Part model, mm, in its own coordinate system. Round coordinates to 2 decimals unless told otherwise and drop trailing zeros. Write each loop counter-clockwise with the first axis right and the second up, starting at its lowest first coordinate (ties: lowest second). Pieces come first, ordered by that corner, then holes. Notation, with made-up numbers: M 12.25,58.25 L 32.25,58.25 A15 cw 32.25,75.25 Z; hole C 60,-17.5 d9. An arc over 180 degrees is marked long. One line per question, with ' | ' between items. Start each with the question number.
1) Saw through at B-B (y = 0). List the corners of the cut face in (x, z).
2) Wall check: probe 1 along Z at (x, y) = (48, 24); probe 2 along X at (y, z) = (42.5, 4.5); probe 3 along X at (y, z) = (0.5, 1.75). Give the ranges that are in metal, low to high. Write a range as [from, to].
3) Drop flat-ended pins along their axis: pin 1 Ø1.5 at (y, z) = (27.5, -1.5) entering from +X; pin 2 Ø1.5 at (y, z) = (-17, 3.5) entering from +X; pin 3 Ø1 at (x, z) = (-48.5, 4) entering from -Y; pin 4 Ø4 at (y, z) = (-36, -1.5) entering from +X. Give the stop position or say it passes through.
4) Saw through at C-C (z = 2.5). List the corners of the cut face in (x, y) (3 decimals), plus the area to 3 significant figures.
5) Saw through at D-D (y = -15.5). List the corners of the cut face in (x, z), plus the area to 3 significant figures.
6) Saw through at A-A (x = 13.5). List the corners of the cut face in (y, z), plus the area to 3 significant figures.
```python
from build123d import *

# Parameters (mm, degrees)
BOSS_EXTRUDE1_DEPTH                               = 6
CSK_FOR_8_FLAT_HEAD_MACHINE_SCREW_100_D           = 4.3053
CSK_FOR_8_FLAT_HEAD_MACHINE_SCREW_100_CSINK_D     = 8.4328
CSK_FOR_8_FLAT_HEAD_MACHINE_SCREW_100_CSINK_ANGLE = 100
SKETCH5_R                                         = 1.905
BOSS_EXTRUDE2_DEPTH                               = 2.5
FILLET1_R                                         = 10
CUT_EXTRUDE1_DEPTH                                = 3.8


with BuildPart() as part:
    # Sketch1 → Boss-Extrude1 (new body)
    with BuildSketch(Plane.XY):
        with BuildLine():
            Line((-26.167728216, 59.5), (26.167728216, 59.5))
            ThreePointArc((26.167728216, 59.5), (65, 0), (26.167728216, -59.5))
            Line((26.167728216, -59.5), (-26.167728216, -59.5))
            ThreePointArc((-26.167728216, -59.5), (-65, 0), (-26.167728216, 59.5))
        make_face()
        with BuildLine():
            Line((-23.650581388, 48.1), (23.650581388, 48.1))
            ThreePointArc((23.650581388, 48.1), (53.6, 0), (23.650581388, -48.1))
            Line((23.650581388, -48.1), (-23.650581388, -48.1))
            ThreePointArc((-23.650581388, -48.1), (-53.6, 0), (-23.650581388, 48.1))
        make_face(mode=Mode.SUBTRACT)
    extrude(amount=BOSS_EXTRUDE1_DEPTH)

    # CSK for #8 Flat Head Machine Screw (100)1 (through all)
    with Locations(Plane.XY.offset(6)):
        with Locations((0, 0), (41.985, 41.985), (-41.985, -41.985), (-41.985, 41.985), (41.985, -41.985)):
            CounterSinkHole(CSK_FOR_8_FLAT_HEAD_MACHINE_SCREW_100_D / 2, CSK_FOR_8_FLAT_HEAD_MACHINE_SCREW_100_CSINK_D / 2, counter_sink_angle=CSK_FOR_8_FLAT_HEAD_MACHINE_SCREW_100_CSINK_ANGLE)

    # Sketch5 → Boss-Extrude2 (add)
    with BuildSketch(Plane(origin=(0, 0, 0), x_dir=(-1, 0, 0), z_dir=(0, 0, -1))):
        with Locations(Location((-59.2455, 0, 0), (0, 0, 180))):
            Circle(SKETCH5_R)
        with Locations(Location((59.2455, 0, 0), (0, 0, 180))):
            Circle(SKETCH5_R)
    extrude(amount=BOSS_EXTRUDE2_DEPTH)

    # Fillet1
    fillet1_edges = [part.edges().sort_by_distance(p)[0] for p in [
        (26.167728216, -59.5, 3),
        (-26.167728216, -59.5, 3),
        (-26.167728216, 59.5, 3),
        (26.167728216, 59.5, 3),
    ]]
    fillet(fillet1_edges, radius=FILLET1_R)

    # Sketch6 → Cut-Extrude1 (cut)
    with BuildSketch(Plane(origin=(0, 0, 0), x_dir=(-1, 0, 0), z_dir=(0, 0, -1))):
        with BuildLine():
            Line((22.912878475, 50), (-22.912878475, 50))
            ThreePointArc((-22.912878475, 50), (-55, 0), (-22.912878475, -50))
            Line((-22.912878475, -50), (22.912878475, -50))
            ThreePointArc((22.912878475, -50), (55, 0), (22.912878475, 50))
        make_face()
    extrude(amount=-CUT_EXTRUDE1_DEPTH, mode=Mode.SUBTRACT)


solid = part.part
```
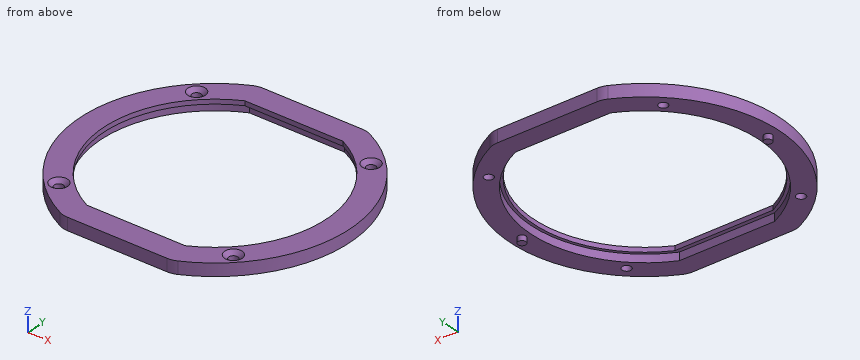
Answer key:
1) outline: M -65,0 L -61.15,0 L -61.15,-2.5 L -57.34,-2.5 L -57.34,0 L -55,0 L -55,3.8 L -53.6,3.8 L -53.6,6 L -65,6 Z; M 53.6,3.8 L 55,3.8 L 55,0 L 57.34,0 L 57.34,-2.5 L 61.15,-2.5 L 61.15,0 L 65,0 L 65,6 L 53.6,6 Z
2) probe 1: z = [3.8, 6] | probe 2: x = [-49.18, -44.36], [-39.61, -32.66], [32.66, 39.61], [44.36, 49.18] | probe 3: x = [-65, -55], [55, 65]
3) pin 1: passes through | pin 2: stops at x = 62.94 | pin 3: stops at y = -43.83 | pin 4: stops at x = 54.98
4) outline: M -28.333,-58.5 A10 ccw -23.974,-59.5 L 23.974,-59.5 A10 ccw 28.333,-58.5 A65 ccw 28.333,58.5 A10 ccw 23.974,59.5 L -23.974,59.5 A10 ccw -28.333,58.5 A65 ccw Z; hole C -41.985,-41.985 d4.305; hole C -41.985,41.985 d4.305; hole M -22.913,-50 L 22.913,-50 A55 ccw 22.913,50 L -22.913,50 A55 ccw Z; hole C 41.985,-41.985 d4.305; hole C 41.985,41.985 d4.305 | area: 3,630 mm2
5) outline: M -63.12,0 L -52.77,0 L -52.77,3.8 L -51.31,3.8 L -51.31,6 L -63.12,6 Z; M 51.31,3.8 L 52.77,3.8 L 52.77,0 L 63.12,0 L 63.12,6 L 51.31,6 Z | area: 131 mm2
6) outline: M -59.5,0 L -50,0 L -50,3.8 L -48.1,3.8 L -48.1,6 L -59.5,6 Z; M 48.1,3.8 L 50,3.8 L 50,0 L 59.5,0 L 59.5,6 L 48.1,6 Z | area: 122 mm2
